Check sheet for the modelled part. Datum: model origin and axes. Units: mm. A direction names the side the tool comes from. Round coordinates to 2 decimals unless told otherwise and drop trailing zeros. Write each loop counter-clockwise with the first axis right and the second up, starting at its lowest first coordinate (ties: lowest second). Pieces come first, ordered by that corner, then holes. Notation, with made-up numbers: (25, 46.5) -> (39, 46.5) arc R18 ccw to (39, 59.5) -> close; hole circle Ø2 at (34, 81.25). An arc over 180 degrees is marked (long way). One line per item, written item: value.
Autodesk Inventor part; units mm, degrees
ref_plane "YZ Plane" through (0, 0, 0) normal (1, 0, 0) x (0, 1, 0)
ref_plane "XZ Plane" through (0, 0, 0) normal (0, 1, 0) x (-1, 0, 0)
ref_plane "XY Plane" through (0, 0, 0) normal (0, 0, 1) x (1, 0, 0)
sketch "Sketch1" plane through (0, 0, 0) normal (0, 0, 1) x (1, 0, 0)
  line L0 (19.05, -19.05) -> (-19.05, -19.05)
  line L1 (-19.05, -19.05) -> (-19.05, 19.05)
  line L2 (-19.05, 19.05) -> (19.05, 19.05)
  line L3 (19.05, 19.05) -> (19.05, -19.05)
  line L4 (19.05, -19.05) -> (-19.05, 19.05) construction
  line L5 (-19.05, -19.05) -> (19.05, 19.05) construction
  line L6 (-19.05, 19.05) -> (19.05, 19.05)
  line L7 (19.05, 19.05) -> (19.05, 44.45)
  line L8 (19.05, 44.45) -> (-19.05, 44.45)
  line L9 (-19.05, 44.45) -> (-19.05, 19.05)
  line L10 (0, 19.05) -> (0, 82.55)
  circle A0 centre (0, 82.55) radius 47.625
  circle A1 centre (0, 82.55) radius 28.575
  point P0 (0, 0)
  dimension "d0" = 38.1
  dimension "d1" = 38.1
  dimension "d2" = 25.4
  dimension "d3" = 63.5
  dimension "d4" = 95.25
  dimension "d5" = 57.15
extrude "Extrusion1" add sketch "Sketch1" along normal blind 6.35
sketch "Sketch2" plane through (0, 0, 6.35) normal (0, 0, 1) x (1, 0, 0)
  circle A0 centre (0, 82.55) radius 28.575 construction
  arc A1 (19.05, 38.901) -> (-19.05, 38.901) centre (0, 82.55) ccw construction
  line L0 (-19.05, 38.901) -> (-19.05, -19.05) construction
  line L1 (-19.05, -19.05) -> (19.05, -19.05) construction
  line L2 (19.05, -19.05) -> (19.05, 38.901) construction
  line L3 (-19.05, -19.05) -> (19.05, -19.05) construction
  line L4 (19.05, -19.05) -> (19.05, 19.05) construction
  line L5 (19.05, 19.05) -> (-19.05, 19.05) construction
  line L6 (-19.05, 19.05) -> (-19.05, -19.05) construction
  line L7 (15.875, -11.43) -> (-15.875, -11.43) construction
  line L8 (-15.875, -11.43) -> (-15.875, 11.43) construction
  line L9 (-15.875, 11.43) -> (15.875, 11.43) construction
  line L10 (15.875, 11.43) -> (15.875, -11.43) construction
  line L11 (15.875, -11.43) -> (-15.875, 11.43) construction
  line L12 (-15.875, -11.43) -> (15.875, 11.43) construction
  line L13 (11.43, -15.875) -> (-11.43, -15.875) construction
  line L14 (-11.43, -15.875) -> (-11.43, 15.875) construction
  line L15 (-11.43, 15.875) -> (11.43, 15.875) construction
  line L16 (11.43, 15.875) -> (11.43, -15.875) construction
  line L17 (11.43, -15.875) -> (-11.43, 15.875) construction
  line L18 (-11.43, -15.875) -> (11.43, 15.875) construction
  line L19 (0, -8.4414) -> (8.4414, 0) construction
  line L20 (8.4414, 0) -> (0, 8.4414) construction
  line L21 (0, 8.4414) -> (-8.4414, 0) construction
  line L22 (-8.4414, 0) -> (0, -8.4414) construction
  line L23 (-5.969, -5.969) -> (5.969, 5.969) construction
  line L24 (5.969, -5.969) -> (-5.969, 5.969) construction
  line L25 (-8.4414, -8.4414) -> (8.4414, -8.4414) construction
  line L26 (8.4414, -8.4414) -> (8.4414, 8.4414) construction
  line L27 (8.4414, 8.4414) -> (-8.4414, 8.4414) construction
  line L28 (-8.4414, 8.4414) -> (-8.4414, -8.4414) construction
  line L29 (-8.4414, -8.4414) -> (8.4414, 8.4414) construction
  line L30 (8.4414, -8.4414) -> (-8.4414, 8.4414) construction
  point P0 (0, 0)
  point P1 (0, 8.4414)
  point P2 (8.4414, 0)
  point P3 (-15.875, 0)
  point P4 (15.875, 0)
  dimension "d8" = 38.1
  dimension "d9" = 38.1
  dimension "d10" = 31.75
  dimension "d11" = 22.86
  dimension "d12" = 22.86
  dimension "d13" = 31.75
  dimension "d14" = 11.938
  dimension "d15" = 11.938
  dimension "d16" = 16.8829
  dimension "d17" = 16.8829
  dimension "d18" = 4.445
  dimension "d19" = 7.4336
  dimension "d20" = 5.969
  dimension "d21" = 5.969
  dimension "d22" = 4.445
  dimension "d23" = 7.4336
  dimension "d24" = 9.906
  dimension "d25" = 9.906
  dimension "d26" = 21.844
  dimension "d27" = 21.844
  dimension "d28" = 3.175
  dimension "d29" = 27.4914
hole "Hole1" at (-15.875, 11.43, 6.35) at (-15.875, 0, 6.35) at (-15.875, -11.43, 6.35) at (15.875, -11.43, 6.35) at (15.875, 0, 6.35) at (15.875, 11.43, 6.35) at (0, 8.4414, 6.35) at (0, -8.4414, 6.35) at (8.4414, 0, 6.35) at (-8.4414, 0, 6.35) direction (0, 0, -1) diameter 3.7973 end through all
properties part number "goniometer_stage_top_v01" material "Stainless Steel AISI 304"
Item 1: Sectioned sample at D-D (x = -20.5). Enter the section's corners in (y, z).
Result set:
outline: (39.56, 0) -> (62.64, 0) -> (62.64, 6.35) -> (39.56, 6.35) -> close; (102.46, 0) -> (125.54, 0) -> (125.54, 6.35) -> (102.46, 6.35) -> close
Item 2: Sectioned sample at C-C (y = 82.55). Enter the section's corners in (x, z) (3 decimals).
Result set:
outline: (-47.625, 0) -> (-28.575, 0) -> (-28.575, 6.35) -> (-47.625, 6.35) -> close; (28.575, 0) -> (47.625, 0) -> (47.625, 6.35) -> (28.575, 6.35) -> close
Item 3: Sectioned sample at B-B (y = 0). Enter the section's corners in (x, z).
Result set:
outline: (-19.05, 0) -> (-17.77, 0) -> (-17.77, 6.35) -> (-19.05, 6.35) -> close; (-13.98, 0) -> (-10.34, 0) -> (-10.34, 6.35) -> (-13.98, 6.35) -> close; (-6.54, 0) -> (6.54, 0) -> (6.54, 6.35) -> (-6.54, 6.35) -> close; (10.34, 0) -> (13.98, 0) -> (13.98, 6.35) -> (10.34, 6.35) -> close; (17.77, 0) -> (19.05, 0) -> (19.05, 6.35) -> (17.77, 6.35) -> close
Item 4: Tool access check on faces 1 (the cylindrical face through (13.993, -11.183, 3.131)), 2 (the flat face through (19.05, 10, 3)), 3 (the flat face through (-19.05, 10, 3)). Record the directions out of +Z, -Z, +X, -X, +Y, -Y that give a thin tool (end or side, any length) a straight path to the whole face; none if there is none.
Result set:
face 1: +Z, -Z
face 2: +Z, -Z, +X, -Y
face 3: +Z, -Z, -X, -Y
Item 5: Depth check by flat-ended pin: pin 1 (6 mm diameter, centred on x = -15.875, y = 0, fed in from +Z); pin 2 (3 mm diameter, centred on y = 11, z = 2, fed in from -X); pin 3 (1.9 mm diameter, centred on y = 3.5, z = 2.5, fed in from +X); pin 4 (1.5 mm diameter, centred on x = 12.5, z = 4, fed in from +Y). Enter the tip coordinate at first touch or a pass-through.
Result set:
pin 1: z = 6.35
pin 2: x = -19.05
pin 3: x = 19.05
pin 4: y = 128.7
Item 6: Sectioned sample at A-A (x = 0). Enter the section's corners in (y, z) (3 decimals).
Result set:
outline: (-19.05, 0) -> (-10.34, 0) -> (-10.34, 6.35) -> (-19.05, 6.35) -> close; (-6.543, 0) -> (6.543, 0) -> (6.543, 6.35) -> (-6.543, 6.35) -> close; (10.34, 0) -> (53.975, 0) -> (53.975, 6.35) -> (10.34, 6.35) -> close; (111.125, 0) -> (130.175, 0) -> (130.175, 6.35) -> (111.125, 6.35) -> close
Item 7: Material ranges on line 1 along Y through (x, z) = (0, 4.5) (3 decimals); line 2 along X through (y, z) = (0, 4.25); line 3 along X through (y, z) = (11.43, 3.25), recorded low to high.
Result set:
line 1: -19.05 to -10.34, -6.543 to 6.543, 10.34 to 53.975, 111.125 to 130.175
line 2: -19.05 to -17.77, -13.98 to -10.34, -6.54 to 6.54, 10.34 to 13.98, 17.77 to 19.05
line 3: -19.05 to -17.77, -13.98 to 13.98, 17.77 to 19.05
